Drawing for the job (mm, zero at the part's lowest x, y, z). Round coordinates to 2 decimals unless told otherwise and drop trailing zeros. Write each loop counter-clockwise with the first axis right and the second up, starting at its lowest first coordinate (ties: lowest second). Pieces come first, ordered by that corner, then holes. Notation, with made-up numbers: (41.25, 2) -> (83.25, 2) arc R25 ccw to (83.25, 19) -> close; hole circle Ø11 at (74, 41.5). An arc over 180 degrees is marked (long way). Answer in a Markdown table with one row per item. Add a question column.
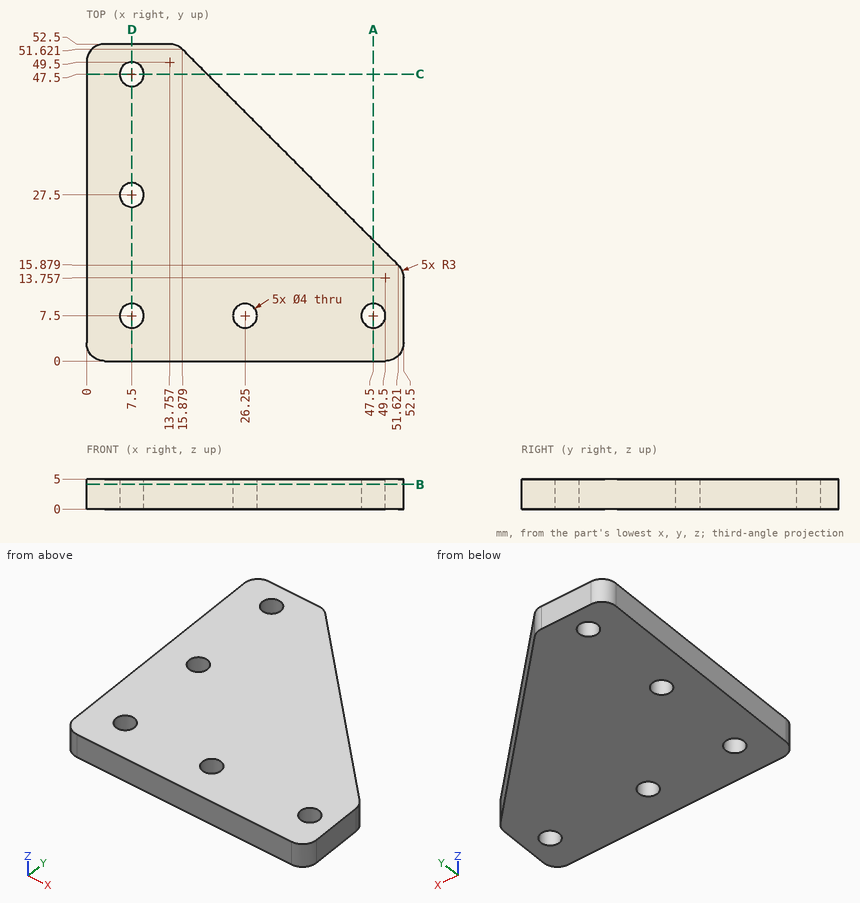
(1) Drop flat-ended pins along their axis: P1, Ø2.5, axis at x = 7.5, y = 47.5, coming from the -Z side; P2, Ø3, axis at x = 26.5, z = 4.5, coming from the +Y side; P3, Ø1.5, axis at y = 46, z = 3.5, coming from the +X side; P4, Ø2, axis at x = 35, z = 3, coming from the +Y side. Give the stop position or say it passes through.
(2) Probe line 1 along Y through (x, z) = (7.5, 2.5); line 2 along X through (y, z) = (8, 0.45); line 3 along Y through (x, z) = (27, 2.2) (1 decimal). List the from-to ranges inside material, lowest first.
(3) Saw through at B-B (z = 4.1). List the corners of the cut face in (x, y), plus the area to 3 significant figures.
(4) Saw through at A-A (x = 47.5). List the corners of the cut face in (y, z), plus the area to 3 significant figures.
(5) Saw through at D-D (x = 7.5). List the corners of the cut face in (y, z).
Answer sheet:
| question | item | result |
|---|---|---|
| 1 | P1 | passes through |
| 1 | P2 | stops at y = 42.5 |
| 1 | P3 | stops at x = 22.25 |
| 1 | P4 | stops at y = 33.5 |
| 2 | line 1 | y = 0 to 5.5, 9.5 to 25.5, 29.5 to 45.5, 49.5 to 52.5 |
| 2 | line 2 | x = 0 to 5.56, 9.44 to 24.31, 28.19 to 45.56, 49.44 to 52.5 |
| 2 | line 3 | y = 0 to 5.6, 9.4 to 40.5 |
| 3 | outline | (0, 3) arc R3 ccw to (3, 0) -> (49.5, 0) arc R3 ccw to (52.5, 3) -> (52.5, 13.76) arc R3 ccw to (51.62, 15.88) -> (15.88, 51.62) arc R3 ccw to (13.76, 52.5) -> (3, 52.5) arc R3 ccw to (0, 49.5) -> close; hole circle Ø4 at (7.5, 7.5); hole circle Ø4 at (7.5, 27.5); hole circle Ø4 at (7.5, 47.5); hole circle Ø4 at (26.25, 7.5); hole circle Ø4 at (47.5, 7.5) |
| 3 | area | 1,980 mm² |
| 4 | outline | (0, 0) -> (5.5, 0) -> (5.5, 5) -> (0, 5) -> close; (9.5, 0) -> (20, 0) -> (20, 5) -> (9.5, 5) -> close |
| 4 | area | 80.0 mm² |
| 5 | outline | (0, 0) -> (5.5, 0) -> (5.5, 5) -> (0, 5) -> close; (9.5, 0) -> (25.5, 0) -> (25.5, 5) -> (9.5, 5) -> close; (29.5, 0) -> (45.5, 0) -> (45.5, 5) -> (29.5, 5) -> close; (49.5, 0) -> (52.5, 0) -> (52.5, 5) -> (49.5, 5) -> close |
